from build123d import *

# Parameters (mm, degrees)
F0_W     = 30
F0_H     = 30
F1_DEPTH = 71.25
F3_DEPTH = 71.251
F4_W     = 5.25
F4_H     = 24
F5_DEPTH = 3.5


# Not quite as in the source:
# - a feature names something its author has since deleted; it is built from what else it names


with BuildPart() as f1:
    # F0 (on Front) → F1 (new body)
    with BuildSketch(Plane.XZ):
        Rectangle(F0_W, F0_H)
    extrude(amount=F1_DEPTH)

    # F2 (on face) → F3 (cut, through all)
    with BuildSketch(Plane.XZ.offset(71.25)):
        with BuildLine():
            Line((6, 9), (6, 15))
            Line((6, 15), (-6, 15))
            Line((-6, 15), (-6, 9))
            ThreePointArc((-6, 9), (0, 3), (6, 9))
        make_face()
    extrude(amount=-F3_DEPTH, mode=Mode.SUBTRACT)

    # F4 (on face) → F5 (cut)
    with BuildSketch(Plane.XZ.offset(71.25)):
        with BuildLine():
            ThreePointArc((-9.75, 9), (-9.2193635213, 12.1726702101), (-7.6852130745, 15))
            Line((-7.6852130745, 15), (-15, 15))
            Line((-15, 15), (-15, 9))
            Line((-15, 9), (-9.75, 9))
        make_face()
        with BuildLine():
            Line((6, 9), (9.75, 9))
            ThreePointArc((9.75, 9), (9.2193635213, 12.1726702101), (7.6852130745, 15))
            Line((7.6852130745, 15), (6, 15))
            Line((6, 15), (6, 9))
        make_face()
        with BuildLine():
            ThreePointArc((7.6852130745, 15), (9.2193635213, 12.1726702101), (9.75, 9))
            Line((9.75, 9), (15, 9))
            Line((15, 9), (15, 15))
            Line((15, 15), (7.6852130745, 15))
        make_face()
        with Locations((-12.375, -3)):
            Rectangle(F4_W, F4_H)
        with Locations((12.375, -3)):
            Rectangle(F4_W, F4_H)
        with BuildLine():
            Line((-6, 15), (-7.6852130745, 15))
            ThreePointArc((-7.6852130745, 15), (-9.2193635213, 12.1726702101), (-9.75, 9))
            Line((-9.75, 9), (-6, 9))
            Line((-6, 9), (-6, 15))
        make_face()
    extrude(amount=-F5_DEPTH, mode=Mode.SUBTRACT)

    # F6: F1 across plane


with BuildPart() as f1_1:
    add(f1.part)
    add(f1.part.mirror(Plane.XZ))


solid = f1_1.part
Verification items for the finished model (mm, model axes). A direction names the side the tool comes from. Give positions to 0.01 mm unless a question says otherwise; leave off trailing zeros. Loops run counter-clockwise (first coordinate to the right, second up) from the corner with the lowest first, then second, coordinate; pieces in that order, holes last.
1) Sectioned sample at C-C, the plane z = -8.25. Enter the section's corners in (x, y).
2) Thickness scan on line 1 along X through (y, z) = (-24, 13.5); line 2 along X through (y, z) = (38, 6.75); line 3 along Z through (x, y) = (-0.25, -29). Record the ranges inside material, lowest first.
3) Set-up check for faces 1 (the flat face through (9.75, -70, -3)), 2 (the flat face through (-6, 1, 12)), 3 (the flat face through (8, 70, 9)): record each of +Z, -Z, +X, -X, +Y, -Y from which the full face is reachable in a straight line by a thin tool's end or side.
4) Depth check by flat-ended pin: pin 1 Ø3 at (y, z) = (-69.5, 1) entering from -X; pin 2 Ø1.8 at (x, y) = (7, -69) entering from +Z; pin 3 Ø6 at (x, y) = (1.5, 30.5) entering from +Z. Enter the tip coordinate at first touch or a pass-through.
5) Sectioned sample at B-B, the plane y = -34. Enter the section's corners in (x, z), then the cut area to 3 significant figures.
6) Draft check along X on faces 4 (the flat face through (8, -70, 9)), 5 (the flat face through (6, 1, 12)), 6 (the flat face through (-9.75, 70, -3)). Enter one of: pulls with the +X half, pulls with the -X half, needs draft (parallel to the pull), parting line crosses it, or undercut.
7) Sectioned sample at A-A, the plane z = 11. Enter the section's corners in (x, y).
8) Sectioned sample at D-D, the plane x = -11.75. Enter the section's corners in (y, z), then the cut area to 4 significant figures.
Answers:
1. outline: (-15, -67.75) - (-9.75, -67.75) - (-9.75, -71.25) - (9.75, -71.25) - (9.75, -67.75) - (15, -67.75) - (15, 67.75) - (9.75, 67.75) - (9.75, 71.25) - (-9.75, 71.25) - (-9.75, 67.75) - (-15, 67.75) - close
2. line 1: x = -15 to -6, 6 to 15
2. line 2: x = -15 to -5.56, 5.56 to 15
2. line 3: z = -15 to 3.01
3. face 1: +Z, -Z, +X, -Y
3. face 2: +Z, +Y, -Y
3. face 3: +Z, +X, -X, +Y
4. pin 1: stops at x = -9.75
4. pin 2: stops at z = 9
4. pin 3: stops at z = 5.03
5. outline: (-15, -15) - (15, -15) - (15, 15) - (6, 15) - (6, 9) arc R6 cw to (-6, 9) - (-6, 15) - (-15, 15) - close
5. area: 771 mm2
6. face 4: needs draft
6. face 5: undercut
6. face 6: pulls with the -X half
7. outline: (-15, -67.75) - (-6, -67.75) - (-6, 67.75) - (-15, 67.75) - close; (6, -67.75) - (15, -67.75) - (15, 67.75) - (6, 67.75) - close
8. outline: (-67.75, -15) - (67.75, -15) - (67.75, 15) - (-67.75, 15) - close
8. area: 4,065 mm2
